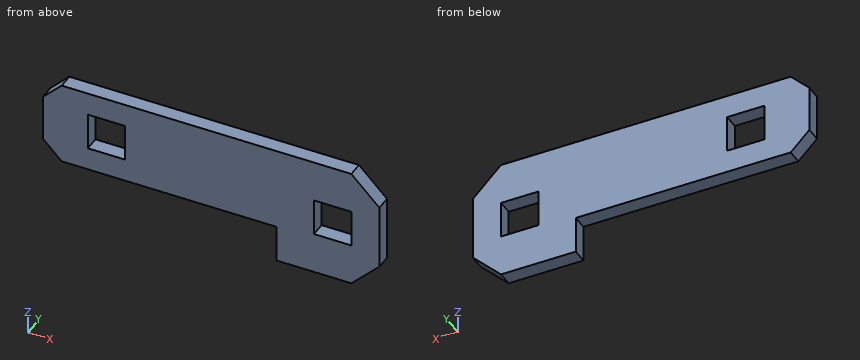
```python
from build123d import *

# Parameters (mm, degrees)
SKETCH_1_W             = 2
SKETCH_1_H             = 2
SM_BASE_FLANGE_1_DEPTH = 0.8
CHAMFER_1_SIZE         = 1
CHAMFER_2_SIZE         = 1.5


# Sheet-metal steps are written as plain solids
with BuildPart() as part:
    # Sketch 1 → Базовая кромка1 (new body)
    with BuildSketch(Plane(origin=(0, 0, 0), x_dir=(1, 0, 0), z_dir=(0, 1, 0))):
        Polygon((0, 0), (0, 4.5), (12.5, 4.5), (12.5, 6.5), (18, 6.5), (18, 0), align=None)
        with Locations((3.4, 2.25)):
            Rectangle(SKETCH_1_W, SKETCH_1_H, mode=Mode.SUBTRACT)
        with Locations((15.5, 3.25)):
            Rectangle(SKETCH_1_W, SKETCH_1_H, mode=Mode.SUBTRACT)
    extrude(amount=-SM_BASE_FLANGE_1_DEPTH)

    # Фаска1
    chamfer_1_edges = [part.edges().sort_by_distance(p)[0] for p in [
        (0, -0.4, 0),
        (0, -0.4, -4.5),
    ]]
    chamfer(chamfer_1_edges, length=CHAMFER_1_SIZE)

    # Фаска2
    chamfer_2_edges = [part.edges().sort_by_distance(p)[0] for p in [
        (18, -0.4, -6.5),
        (18, -0.4, 0),
    ]]
    chamfer(chamfer_2_edges, length=CHAMFER_2_SIZE)


solid = part.part
```
Read the model definition and answer for the solid it produces. Units are mm, in the model's axes. Coordinates: 2 decimals unless noted, no trailing zeros. Write each loop counter-clockwise with the first axis right and the second up, starting at its lowest first coordinate (ties: lowest second). Pieces come first, ordered by that corner, then holes. Notation, with made-up numbers: (39, 85) -> (96, 85) arc R19 ccw to (96, 102) -> close; hole circle Ø4 at (57, 55). An arc over 180 degrees is marked (long way). Answer as a JSON object with one key per item and string values.
Q1. The part is cut by section B-B on x = 16. Give the vertices of the cut face in (y, z).
The answers:
{"outline": "(-0.8, -6.5) -> (0, -6.5) -> (0, -4.25) -> (-0.8, -4.25) -> close; (-0.8, -2.25) -> (0, -2.25) -> (0, 0) -> (-0.8, 0) -> close"}
Q2. The part is cut by section D-D on z = -2. Give the vertices of the cut face in (x, y).
The answers:
{"outline": "(0, -0.8) -> (2.4, -0.8) -> (2.4, 0) -> (0, 0) -> close; (4.4, -0.8) -> (18, -0.8) -> (18, 0) -> (4.4, 0) -> close"}
Q3. The part is cut by section C-C on z = -3. Give the vertices of the cut face in (x, y), then the cut area to 3 significant figures.
The answers:
{"outline": "(0, -0.8) -> (2.4, -0.8) -> (2.4, 0) -> (0, 0) -> close; (4.4, -0.8) -> (14.5, -0.8) -> (14.5, 0) -> (4.4, 0) -> close; (16.5, -0.8) -> (18, -0.8) -> (18, 0) -> (16.5, 0) -> close", "area": "11.2 mm2"}
Q4. The part is cut by section A-A on y = -0.3. Give the vertices of the cut face in (x, z), then the cut area to 4 significant figures.
The answers:
{"outline": "(0, -3.5) -> (1, -4.5) -> (12.5, -4.5) -> (12.5, -6.5) -> (16.5, -6.5) -> (18, -5) -> (18, -1.5) -> (16.5, 0) -> (1, 0) -> (0, -1) -> close; hole (2.4, -3.25) -> (4.4, -3.25) -> (4.4, -1.25) -> (2.4, -1.25) -> close; hole (14.5, -4.25) -> (16.5, -4.25) -> (16.5, -2.25) -> (14.5, -2.25) -> close", "area": "80.75 mm2"}
Q5. Consider line 1 (X direction, y = -0.55, z = -2.75); line 2 (Z direction, x = 16, y = -0.25); line 3 (X direction, y = -0.1, z = -2). Determine where each line is inside the solid, lowest interval first. Write a range as [from, to].
The answers:
{"line 1": "x = [0, 2.4], [4.4, 14.5], [16.5, 18]", "line 2": "z = [-6.5, -4.25], [-2.25, 0]", "line 3": "x = [0, 2.4], [4.4, 18]"}
